Could you check a few things on this model? Use its own coordinates, in mm. Coordinates: 2 decimals unless noted, no trailing zeros. Order: outer loops, then holes, each group sorted by start corner. A loop starts at its lowest first (then second) coordinate and runs counter-clockwise, first axis right, second up. Notation, with made-up numbers: (8.25, 87.5) - (51.25, 87.5) arc R11 ccw to (51.25, 107.5) - close; hole circle Ø10 at (-25.5, -25.5). An arc over 180 degrees is marked (long way). One line per item, written item: value.
from build123d import *

# Parameters (mm, degrees)
SKETCH_1_W      = 80
SKETCH_1_H      = 50
SKETCH_1_R      = 10
EXTRUDE_1_DEPTH = 25


with BuildPart() as part:
    # Эскиз1 → Бобышка-Вытянуть1 (new body, symmetric)
    with BuildSketch(Plane.XY):
        with Locations((10, 0)):
            Rectangle(SKETCH_1_W, SKETCH_1_H)
        Circle(SKETCH_1_R, mode=Mode.SUBTRACT)
    extrude(amount=EXTRUDE_1_DEPTH, both=True)


solid = part.part
Item 1: I want a section at A-A on y = -8. Please give me the cut outline in (x, z), then the cut area to 3 significant figures.
Conclusion:
outline: (-30, -25) - (-6, -25) - (-6, 25) - (-30, 25) - close; (6, -25) - (50, -25) - (50, 25) - (6, 25) - close
area: 3,400 mm²
Item 2: I want a section at B-B on x = 0. Please give me the cut outline in (y, z).
Conclusion:
outline: (-25, -25) - (-10, -25) - (-10, 25) - (-25, 25) - close; (10, -25) - (25, -25) - (25, 25) - (10, 25) - close
Item 3: Thinking about a two-plate mould opening in X: for faces 1 (the face through (9, 25, 0)), 2 (the face through (-30, 0, 0)), 3 (the face through (-2.17, -9.76, -0.35)), which applies, pulls with the +X half, pulls with the -X half, needs draft (parallel to the pull), parting line crosses it, or undercut?
Conclusion:
face 1: needs draft
face 2: pulls with the -X half
face 3: undercut
Item 4: If I drill on probe 1 along Y at (x, z) = (0, 11); probe 2 along X at (y, z) = (-9, -12); probe 3 along X at (y, z) = (2, 0), over which ranges is the centre line in solid material (lowest first)?
Conclusion:
probe 1: -25 to -10, 10 to 25
probe 2: -30 to -4.36, 4.36 to 50
probe 3: -30 to -9.8, 9.8 to 50
Item 5: I'm going to push a flat-ended pin straight in: pin 1 Ø18 at (x, y) = (0, 0) entering from -Z. Where does the tip first touch, or does it pass through?
Conclusion:
pin 1: through
Item 6: I want a section at C-C on z = 8. Please give me the cut outline in (x, y), then the cut area to 3 significant figures.
Conclusion:
outline: (-30, -25) - (50, -25) - (50, 25) - (-30, 25) - close; hole circle Ø20 at (0, 0)
area: 3,690 mm²
